from build123d import *

# Parameters (mm, degrees)
BOSS_EXTRUDE2_DEPTH      = 12.5
SKETCH7_W                = 4
SKETCH7_H                = 2
CUT_EXTRUDE10_DEPTH      = 26
CUT_EXTRUDE11_DEPTH      = 4
CUT_EXTRUDE11_DEPTH_BACK = 10.5


with BuildPart() as part:
    # Sketch1 → Boss-Extrude2 (new body)
    with BuildSketch(Plane.XY):
        Polygon((-90.614577373, 45.459408198), (-87.614577373, 45.459408198), (-87.614577373, 42.459408198), (-83.614577373, 42.459408198), (-83.614577373, 45.459408198), (-79.614577373, 45.459408198), (-79.614577373, 32.959408198), (-83.614577373, 32.959408198), (-83.614577373, 35.959408198), (-87.614577373, 35.959408198), (-87.614577373, 32.959408198), (-90.614577373, 32.959408198), align=None)
    extrude(amount=BOSS_EXTRUDE2_DEPTH)

    # Sketch7 → Cut-Extrude10 (cut)
    with BuildSketch(Plane(origin=(0, 42.459408198, 0), x_dir=(1, 0, 0), z_dir=(0, 1, 0))):
        with Locations((-85.614577373, -11.5)):
            Rectangle(SKETCH7_W, SKETCH7_H)
    extrude(amount=-CUT_EXTRUDE10_DEPTH, mode=Mode.SUBTRACT)

    # Sketch8 → Cut-Extrude11 (cut, two sides)
    with BuildSketch(Plane(origin=(0, 42.459408198, 0), x_dir=(1, 0, 0), z_dir=(0, 1, 0))) as cut_extrude11_sk:
        Polygon((-87.614577373, 39.681644159), (-87.614577373, 0), (-87.614577373, -2), (-83.614577373, -2), (-83.614577373, 0), (-83.614577373, 39.681644159), (-83.614577373, 119.044932478), (-87.614577373, 119.044932478), align=None)
    extrude(amount=CUT_EXTRUDE11_DEPTH, mode=Mode.SUBTRACT)
    extrude(cut_extrude11_sk.sketch, amount=-CUT_EXTRUDE11_DEPTH_BACK, mode=Mode.SUBTRACT)


solid = part.part
Geometry: final body of the model. Coordinates: model frame, mm. A direction names the side the tool comes from. Give positions to 0.01 mm unless a question says otherwise; leave off trailing zeros. Write each loop counter-clockwise with the first axis right and the second up, starting at its lowest first coordinate (ties: lowest second). Pieces come first, ordered by that corner, then holes.
(1) Mould query, pull axis X, two halves, no side actions, for faces 1 (the flat face through (-87.615, 35, 6)), 2 (the flat face through (-82, 39, 12.5)), 3 (the flat face through (-79.615, 39, 6)). Classes: released by +X, released by -X, zero draft, split by the parting line, or undercut.
(2) Ray query, line 1 (X direction, y = 40.75, z = 0.5); line 2 (Y direction, x = -85, z = 4.5); line 3 (Z direction, x = -84, y = 37.5). Return the intervals inside material, ascending.
(3) Access query for faces 4 (the flat face through (-86, 39, 2)), 5 (the flat face through (-86, 42.459, 6)), 6 (the flat face through (-86, 39, 10.5)), 7 (the flat face through (-86, 35.959, 6)). Directions: +Z, -Z, +X, -X, +Y, -Y. A direction counts if a zero-diameter tool reaches every point of the face in a straight line with its end or side. Return the directions, or none.
(4) First-contact query: P1, Ø1.5, axis at x = -85, z = 6.5, coming from the -Y side; P2, Ø2, axis at x = -85, y = 39, coming from the -Z side; P3, Ø3, axis at x = -86, y = 39, coming from the +Z side. Flat tips, straight axial feed; report the tip coordinate or a pass-through.
(5) Cut plane D-D, the plane x = -85. Return loops of the section in (y, z).
(6) Cut plane A-A, the plane z = 11.5. Return loops of the section in (x, y), then the cut area to 3 significant figures.
(7) Cut plane C-C, the plane z = 4. Return loops of the section in (x, y).
(8) Cut plane B-B, the plane y = 35.75. Return loops of the section in (x, z), then the cut area to 3 significant figures.
Values follow:
1. face 1: undercut
1. face 2: zero draft
1. face 3: released by +X
2. line 1: x = -90.61 to -87.61, -83.61 to -79.61
2. line 2: y = 35.96 to 42.46
2. line 3: z = 2 to 10.5
3. face 4: -Z, +Y, -Y
3. face 5: +Z, -Z, +Y
3. face 6: +Z, +Y, -Y
3. face 7: +Z, -Z, -Y
4. P1: stops at y = 35.96
4. P2: stops at z = 2
4. P3: stops at z = 10.5
5. outline: (35.96, 2) - (42.46, 2) - (42.46, 10.5) - (35.96, 10.5) - close
6. outline: (-90.61, 32.96) - (-87.61, 32.96) - (-87.61, 45.46) - (-90.61, 45.46) - close; (-83.61, 32.96) - (-79.61, 32.96) - (-79.61, 45.46) - (-83.61, 45.46) - close
6. area: 87.5 mm2
7. outline: (-90.61, 32.96) - (-87.61, 32.96) - (-87.61, 35.96) - (-83.61, 35.96) - (-83.61, 32.96) - (-79.61, 32.96) - (-79.61, 45.46) - (-83.61, 45.46) - (-83.61, 42.46) - (-87.61, 42.46) - (-87.61, 45.46) - (-90.61, 45.46) - close
8. outline: (-90.61, 0) - (-87.61, 0) - (-87.61, 12.5) - (-90.61, 12.5) - close; (-83.61, 0) - (-79.61, 0) - (-79.61, 12.5) - (-83.61, 12.5) - close
8. area: 87.5 mm2
